Design review of the part shown in the three views and the two pictorial views. Dimensions are in mm from the part's minimum x, y and z. A direction names the side the tool comes from. Round coordinates to 2 decimals unless told otherwise and drop trailing zeros. Order: outer loops, then holes, each group sorted by start corner. A loop starts at its lowest first (then second) coordinate and runs counter-clockwise, first axis right, second up.
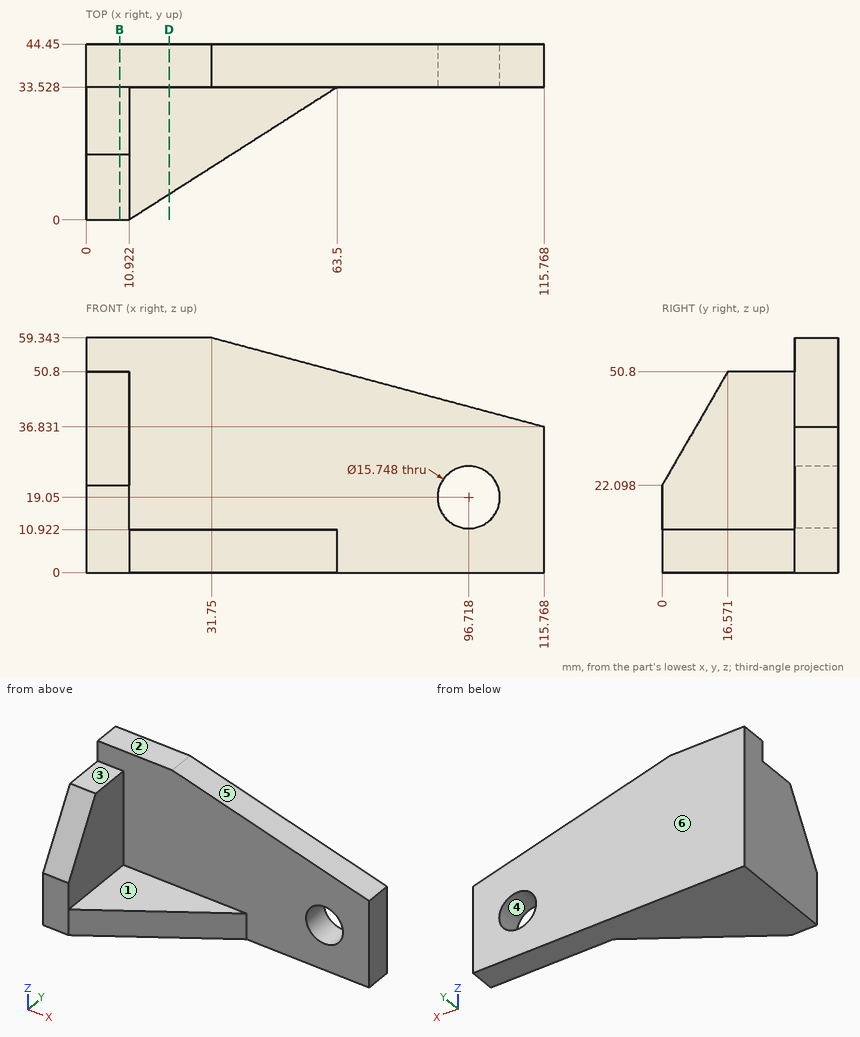
(1) Draft analysis for pull direction Z (two halves, no side actions). For the marked faces 4, 5 and 6, state which applies: pulls with the +Z half, pulls with the -Z half, needs draft (parallel to the pull), parting line crosses it, or undercut.
Data:
face 4: undercut
face 5: pulls with the +Z half
face 6: needs draft
(2) Consider section D-D (x = 21). Write out the cut boundary in (y, z), and give its area (3 significant figures).
Data:
outline: (6.43, 0) - (44.45, 0) - (44.45, 59.34) - (33.53, 59.34) - (33.53, 10.92) - (6.43, 10.92) - close
area: 944 mm2
(3) Consider section B-B (x = 8.5). Write out the cut boundary in (y, z), and give its area (3 significant figures).
Data:
outline: (0, 0) - (44.45, 0) - (44.45, 59.34) - (33.53, 59.34) - (33.53, 50.8) - (16.57, 50.8) - (0, 22.1) - close
area: 2,110 mm2
(4) To check wall thickness, follow probe 1 along X at (y, z) = (40, 19) (1 decimal); probe 2 along X at (y, z) = (5, 14); probe 3 along Y at (x, z) = (54, 33). State the ranges of each line that lie inside material, in increasing order.
Data:
probe 1: x = 0 to 88.8, 104.6 to 115.8
probe 2: x = 0 to 10.92
probe 3: y = 33.53 to 44.45
(5) For the marked faces 1, 2 and 3, list the 3-axis set-ups (+Z, -Z, +X, -X, +Y, -Y) from which the entire face can be reached by the end or side of a thin tool; tool diameter is ignored.
Data:
face 1: +Z, +X, -Y
face 2: +Z, +X, -X, +Y, -Y
face 3: +Z, +X, -X, -Y
(6) Insertion check: pin 1 (10 mm diameter, centred on y = 10.5, z = 28, fed in from +X); pin 2 (10 mm diameter, centred on x = 27.5, y = 16, fed in from +Z); pin 3 (8.5 mm diameter, centred on x = 8, y = 28, fed in from +Z); pin 4 (10 mm diameter, centred on y = 37, z = 35.5, fed in from -X). Each pin has a flat end and moves straight along its axis. Give the tip position at first contact, or say it passes through.
Data:
pin 1: stops at x = 10.92
pin 2: stops at z = 10.92
pin 3: stops at z = 50.8
pin 4: stops at x = 0
